from build123d import *

# Parameters (mm, degrees)
SKETCH1_R                      = 3.5
BOSS_EXTRUDE1_DEPTH            = 0.75
F_2_2_2_2_DIAMETER_HOLE1_D     = 2.2
F_3_2_3_2_DIAMETER_HOLE1_D     = 3.2
F_3_2_3_2_DIAMETER_HOLE1_DEPTH = 10
F_3_2_3_2_DIAMETER_HOLE1_TIP   = 0.96137699
CUT_EXTRUDE1_DEPTH             = 128.152713302
FILLET1_R                      = 2
SKETCH7_R                      = 4
CUT_EXTRUDE2_DEPTH             = 128.15271342
CUT_EXTRUDE3_DEPTH             = 5


with BuildPart() as part:
    # Sketch1 → Boss-Extrude1 (new, symmetric)
    with BuildSketch(Plane(origin=(0, 0, 0), x_dir=(1, 0, 0), z_dir=(0, 1, 0))):
        with BuildLine():
            ThreePointArc((-37.239092363, -21.5), (-43, 0), (-37.239092363, 21.5))
            ThreePointArc((-37.239092363, 21.5), (-36.567343094, 22.335249783), (-35.674318722, 22.928037055))
            ThreePointArc((-35.674318722, 22.928037055), (-69.961373448, 13.496685886), (-105.45946442, 15.603352454))
            ThreePointArc((-105.45946442, 15.603352454), (-125, 0), (-105.45946442, -15.603352454))
            ThreePointArc((-105.45946442, -15.603352454), (-69.961373448, -13.496685886), (-35.674318722, -22.928037055))
            ThreePointArc((-35.674318722, -22.928037055), (-36.567343094, -22.335249783), (-37.239092363, -21.5))
        make_face()
        with BuildLine():
            ThreePointArc((-31.176914536, 18), (-35.958003449, 16.718911087), (-37.239092363, 21.5))
            ThreePointArc((-37.239092363, 21.5), (-43, 0), (-37.239092363, -21.5))
            ThreePointArc((-37.239092363, -21.5), (-35.958003449, -16.718911087), (-31.176914536, -18))
            ThreePointArc((-31.176914536, -18), (-36, 0), (-31.176914536, 18))
        make_face()
        with Locations((-34.208003449, -19.75)):
            Circle(SKETCH1_R)
        with Locations((-34.208003449, 19.75)):
            Circle(SKETCH1_R)
    extrude(amount=BOSS_EXTRUDE1_DEPTH, both=True)

    # Ø2.2 (2.2) Diameter Hole1 (through all)
    with Locations(Plane(origin=(0, 0.75, 0), x_dir=(1, 0, 0), z_dir=(0, 1, 0))):
        with Locations((-114.480077554, 5.480077554), (-103.519922446, 5.480077554), (-103.519922446, -5.480077554), (-114.480077554, -5.480077554)):
            Hole(F_2_2_2_2_DIAMETER_HOLE1_D / 2)

    # Ø3.2 (3.2) Diameter Hole1
    with Locations(Plane(origin=(0, 0.75, 0), x_dir=(1, 0, 0), z_dir=(0, 1, 0))):
        with Locations((-34.208003449, 19.75), (-34.208003449, -19.75), (-92.21668251, 9.928255337), (-92.21668251, -9.928255337)):
            Hole(F_3_2_3_2_DIAMETER_HOLE1_D / 2, depth=F_3_2_3_2_DIAMETER_HOLE1_DEPTH)
            with Locations((0, 0, -(F_3_2_3_2_DIAMETER_HOLE1_DEPTH + F_3_2_3_2_DIAMETER_HOLE1_TIP / 2))):  # 118° drill point
                Cone(0, F_3_2_3_2_DIAMETER_HOLE1_D / 2, F_3_2_3_2_DIAMETER_HOLE1_TIP, mode=Mode.SUBTRACT)

    # Sketch6 → Cut-Extrude1 (cut, through all)
    with BuildSketch(Plane(origin=(0, 0.75, 0), x_dir=(1, 0, 0), z_dir=(0, 1, 0))):
        with BuildLine():
            Line((-69.980899838, -6.458648161), (-46.735459102, 0))
            Line((-46.735459102, 0), (-69.980899838, 6.458648161))
            ThreePointArc((-69.980899838, 6.458648161), (-82.217649484, 5.904514504), (-94.444607799, 6.643836082))
            ThreePointArc((-94.444607799, 6.643836082), (-93, 0), (-94.444607799, -6.643836082))
            ThreePointArc((-94.444607799, -6.643836082), (-82.217649484, -5.904514504), (-69.980899838, -6.458648161))
        make_face()
        with BuildLine():
            Line((-64.779742297, 7.089291637), (-42.987555952, 1.03442411))
            ThreePointArc((-42.987555952, 1.03442411), (-42.397380289, 7.173712054), (-40.934970503, 13.165416435))
            ThreePointArc((-40.934970503, 13.165416435), (-52.695786799, 9.493300195), (-64.779742297, 7.089291637))
        make_face()
        with BuildLine():
            ThreePointArc((-40.934970503, -13.165416435), (-42.397380289, -7.173712054), (-42.987555952, -1.03442411))
            Line((-42.987555952, -1.03442411), (-64.779742297, -7.089291637))
            ThreePointArc((-64.779742297, -7.089291637), (-52.695786799, -9.493300195), (-40.934970503, -13.165416435))
        make_face()
    extrude(amount=-CUT_EXTRUDE1_DEPTH, mode=Mode.SUBTRACT)

    # Fillet1
    fillet1_edges = [part.edges().sort_by_distance(p)[0] for p in [
        (-42.987555952, 0, 1.03442411),
        (-40.934970503, 0, 13.165416435),
        (-64.779742297, 0, 7.089291637),
        (-94.444607799, 0, 6.643836082),
        (-94.444607799, 0, -6.643836082),
        (-69.980899838, 0, -6.458648161),
        (-46.735459102, 0, 0),
        (-69.980899838, 0, 6.458648161),
        (-40.934970503, 0, -13.165416435),
        (-42.987555952, 0, -1.03442411),
        (-64.779742297, 0, -7.089291637),
    ]]
    fillet(fillet1_edges, radius=FILLET1_R)

    # Sketch7 → Cut-Extrude2 (cut, through all)
    with BuildSketch(Plane(origin=(0, 0.75, 0), x_dir=(1, 0, 0), z_dir=(0, 1, 0))):
        with Locations(Location((-109, 0, 0), (0, 0, 270))):
            Circle(SKETCH7_R)
    extrude(amount=-CUT_EXTRUDE2_DEPTH, mode=Mode.SUBTRACT)

    # Sketch8 → Cut-Extrude3 (cut, symmetric)
    with BuildSketch(Plane(origin=(0, 0.75, 0), x_dir=(1, 0, 0), z_dir=(0, 1, 0))):
        with BuildLine():
            ThreePointArc((-99.206571081, 8.237794001), (-99.206571081, 9.793428919), (-100.762205999, 9.793428919))
            Line((-100.762205999, 9.793428919), (-104.297739905, 6.257895014))
            ThreePointArc((-104.297739905, 6.257895014), (-103.09897067, 6.49634504), (-102.419922446, 5.480077554))
            ThreePointArc((-102.419922446, 5.480077554), (-102.50365496, 5.059125779), (-102.742104986, 4.702260095))
            Line((-102.742104986, 4.702260095), (-99.206571081, 8.237794001))
        make_face()
        with BuildLine():
            ThreePointArc((-100.762205999, -9.793428919), (-99.206571081, -9.793428919), (-99.206571081, -8.237794001))
            Line((-99.206571081, -8.237794001), (-102.742104986, -4.702260095))
            ThreePointArc((-102.742104986, -4.702260095), (-102.50365496, -5.059125779), (-102.419922446, -5.480077554))
            ThreePointArc((-102.419922446, -5.480077554), (-103.09897067, -6.49634504), (-104.297739905, -6.257895014))
            Line((-104.297739905, -6.257895014), (-100.762205999, -9.793428919))
        make_face()
        with BuildLine():
            Line((-115.257895014, -4.702260095), (-118.793428919, -8.237794001))
            ThreePointArc((-118.793428919, -8.237794001), (-118.793428919, -9.793428919), (-117.237794001, -9.793428919))
            Line((-117.237794001, -9.793428919), (-113.702260095, -6.257895014))
            ThreePointArc((-113.702260095, -6.257895014), (-115.257895014, -6.257895014), (-115.257895014, -4.702260095))
        make_face()
        with BuildLine():
            Line((-113.702260095, 6.257895014), (-117.237794001, 9.793428919))
            ThreePointArc((-117.237794001, 9.793428919), (-118.793428919, 9.793428919), (-118.793428919, 8.237794001))
            Line((-118.793428919, 8.237794001), (-115.257895014, 4.702260095))
            ThreePointArc((-115.257895014, 4.702260095), (-115.257895014, 6.257895014), (-113.702260095, 6.257895014))
        make_face()
    extrude(amount=CUT_EXTRUDE3_DEPTH, both=True, mode=Mode.SUBTRACT)


solid = part.part
Work out the finished part from the listing and answer in its coordinate system (mm). Round coordinates to 2 decimals unless told otherwise and drop trailing zeros. Write each loop counter-clockwise with the first axis right and the second up, starting at its lowest first coordinate (ties: lowest second). Pieces come first, ordered by that corner, then holes. Notation, with made-up numbers: (69, 74) -> (106, 74) arc R37 ccw to (106, 113) -> close; hole circle Ø1 at (1, 15.25). An arc over 180 degrees is marked (long way). Write each question's results on one line, items separated by ' | '.
Item 1: A cutting plane is placed at A-A, the plane z = 0. Determine the outline of the cut face in (x, y).
Result set:
outline: (-125, -0.75) -> (-113, -0.75) -> (-113, 0.75) -> (-125, 0.75) -> close; (-105, -0.75) -> (-93, -0.75) -> (-93, 0.75) -> (-105, 0.75) -> close; (-52.21, -0.75) -> (-36, -0.75) -> (-36, 0.75) -> (-52.21, 0.75) -> close
Item 2: A cutting plane is placed at D-D, the plane x = -48. Determine the outline of the cut face in (y, z), plus the area to 3 significant figures.
Result set:
outline: (-0.75, -18.13) -> (0.75, -18.13) -> (0.75, -10.8) -> (-0.75, -10.8) -> close; (-0.75, -2.43) -> (0.75, -2.43) -> (0.75, 2.43) -> (-0.75, 2.43) -> close; (-0.75, 10.8) -> (0.75, 10.8) -> (0.75, 18.13) -> (-0.75, 18.13) -> close | area: 29.3 mm^2
Item 3: The mould has two halves that part along Z. Classify faces 1 (the face through (-70.459, 0.01, 13.446)), 2 (the face through (-100.95, -0.01, 6.495)): +Z half, -Z half, draft (parallel to the pull), parting line (faces both ways), or undercut.
Result set:
face 1: +Z half | face 2: undercut
Item 4: A cutting plane is placed at B-B, the plane x = -83.5. Determine the outline of the cut face in (y, z).
Result set:
outline: (-0.75, -12.92) -> (0.75, -12.92) -> (0.75, -5.92) -> (-0.75, -5.92) -> close; (-0.75, 5.92) -> (0.75, 5.92) -> (0.75, 12.92) -> (-0.75, 12.92) -> close
Item 5: Find the intervals of material crossed by line 1 along Z through (x, y) = (-56, -0.3); line 2 along Z through (x, y) = (-103.5, -0.1); line 3 along Z through (x, y) = (-51.5, -0.2), in increasing order. Write a range as [from, to].
Result set:
line 1: [-15.89, -8.7], [-4.65, -2.57], [2.57, 4.65], [8.7, 15.89] | line 2: [-15.18, -7.06], [-4.38, 4.38], [7.06, 15.18] | line 3: [-17.07, -9.8], [-3.4, 3.4], [9.8, 17.07]
Item 6: A cutting plane is placed at C-C, the plane z = 14.5. Determine the outline of the cut face in (x, y), plus the area to 3 significant figures.
Result set:
outline: (-115.76, -0.75) -> (-99.94, -0.75) -> (-99.94, 0.75) -> (-115.76, 0.75) -> close; (-62.74, -0.75) -> (-32.95, -0.75) -> (-32.95, 0.75) -> (-62.74, 0.75) -> close | area: 68.4 mm^2
